```python
from build123d import *

# Parameters (mm, degrees)
SKETCH1_R           = 6.625
SKETCH1_R_2         = 6.307204498
BOSS_EXTRUDE1_DEPTH = 27
SKETCH1_3_R         = 6.307204498
BOSS_EXTRUDE2_DEPTH = 38
SKETCH2_R           = 5.925018159
BOSS_EXTRUDE3_DEPTH = 9


with BuildPart() as part:
    # Sketch1 → Boss-Extrude1 (new body)
    # profile 1 of 2: a face of its own
    with BuildSketch(Plane.XY):
        Circle(SKETCH1_R)
        Circle(SKETCH1_R_2, mode=Mode.SUBTRACT)
    # profile 2 of 2: a face of its own
    with BuildSketch(Plane.XY):
        Circle(SKETCH1_R_2)
    extrude(amount=BOSS_EXTRUDE1_DEPTH)

    # Sketch1_3 → Boss-Extrude2 (add)
    with BuildSketch(Plane.XY):
        Circle(SKETCH1_3_R)
    extrude(amount=BOSS_EXTRUDE2_DEPTH)

    # Sketch2 → Boss-Extrude3 (add)
    with BuildSketch(Plane.XY.offset(38)):
        Circle(SKETCH2_R)
    extrude(amount=BOSS_EXTRUDE3_DEPTH)


solid = part.part
```
Model file for the job. Use its own axes, mm. A direction names the side the tool comes from. Coordinates: 2 decimals unless noted, no trailing zeros. Write each loop counter-clockwise with the first axis right and the second up, starting at its lowest first coordinate (ties: lowest second). Pieces come first, ordered by that corner, then holes. Notation, with made-up numbers: (5, -18) - (10, -18) arc R12 ccw to (10, -13) - close; hole circle Ø7 at (-39, 60.5). An arc over 180 degrees is marked (long way). One line per question, with ' | ' between items. Start each with the question number.
Q1. Cut at D-D, the plane z = 25. List the corners of the cut face in (x, y) (3 decimals).
Q2. Cut at A-A, the plane x = 0. List the corners of the cut face in (y, z) (3 decimals).
Q3. Drill centre lines: line 1 (Z direction, x = 5, y = 4.25); line 2 (Z direction, x = -5, y = 3.5); line 3 (X direction, y = 0.25, z = 34). Where is each one in solid material? Low to high. Write a range as [from, to].
Q4. Cut at C-C, the plane z = 43. List the corners of the cut face in (x, y), then the cut area to 3 significant figures.
Q5. 3-axis set-ups, long thin cutter, end or side, ignore diameter. For faces 1 (the face through (-1.367, -6.157, 32.423)), 2 (the face through (0, 0, 47)): which of +Z, -Z, +X, -X, +Y, -Y reach the whole face in a straight line?
Q6. Pin check, flat tips, straight feed: pin 1 (1.5 mm diameter, centred on x = -5, z = 32.5, fed in from -Y); pin 2 (3 mm diameter, centred on y = 2, z = 26.5, fed in from -X); pin 3 (5 mm diameter, centred on x = 3.5, z = 17.5, fed in from +Y). Stop position of each tip, or through.
Answer below:
1) outline: circle Ø13.25 at (0, 0)
2) outline: (-6.625, 0) - (6.625, 0) - (6.625, 27) - (6.307, 27) - (6.307, 38) - (5.925, 38) - (5.925, 47) - (-5.925, 47) - (-5.925, 38) - (-6.307, 38) - (-6.307, 27) - (-6.625, 27) - close
3) line 1: [0, 27] | line 2: [0, 38] | line 3: [-6.3, 6.3]
4) outline: circle Ø11.85 at (0, 0) | area: 110 mm^2
5) face 1: +Z | face 2: +Z, +X, -X, +Y, -Y
6) pin 1: y = -4.66 | pin 2: x = -6.61 | pin 3: y = 6.55
